Part model, mm, in its own coordinate system. Face numbers are marked on the shaded views. A direction names the side the tool comes from. Give positions to 0.01 mm unless a question says otherwise; leave off trailing zeros. Write each loop counter-clockwise with the first axis right and the second up, starting at its lowest first coordinate (ties: lowest second). Pieces come first, ordered by that corner, then holes. Notation, with made-up numbers: M 63.25,-18 L 74.25,-18 A24 cw 74.25,17 Z; hole C 46,9.25 d4. An arc over 180 degrees is marked long. Use CSV: the item, a comma, the result in double quotes. Start each with the question number.
Item 1: Cut at C-C (x = -6). List the corners of the cut face in (y, z) (3 decimals), then the cut area to 3 significant figures.
Item 2: Cut at A-A (y = 9.5). List the corners of the cut face in (x, z) (3 decimals), then the cut area to 3 significant figures.
Item 3: Cut at B-B (z = 0.6). List the corners of the cut face in (x, y) (3 decimals), then the cut area to 3 significant figures.
Item 4: Drill centre lines: line 1 (X direction, y = 2, z = 1.7) (3 decimals); line 2 (Y direction, x = 1.5, z = 0.6) (3 decimals). Where is each one in solid material? Low to high. Write a range as [from, to].
Item 5: Which spindle directions (+Z, -Z, +X, -X, +Y, -Y) get a long thin tool onto all of the face, cutting with end or side? Do the marked faces 1 and 2. Say none if no direction does.
Item 6: Pin check, flat tip, straight feed: pin 1 (0.9 mm diameter, centred on x = 5.5, z = 2.5, fed in from +Y) (3 decimals). Stop position of the tip, or through.
from build123d import *

# Parameters (mm, degrees)
F0_W     = 36.83
F0_H     = 36.83
F1_DEPTH = 3.1496
F2_W     = 31.75
F2_H     = 31.75
F3_DEPTH = 25.4
F4_W     = 31.75
F4_H     = 2.54
F5_DEPTH = 25.4


with BuildPart() as f1:
    # F0 (on Top) → F1 (new body)
    with BuildSketch(Plane.XY):
        Rectangle(F0_W, F0_H)
    extrude(amount=F1_DEPTH)

    # F2 (on face) → F3 (cut)
    with BuildSketch(Plane.XY.offset(3.1496)):
        Rectangle(F2_W, F2_H)
    extrude(amount=-F3_DEPTH, mode=Mode.SUBTRACT)

    # F4 (on face) → F5 (cut)
    with BuildSketch(Plane.XY.offset(3.1496)):
        with Locations((0, 17.145)):
            Rectangle(F4_W, F4_H)
    extrude(amount=-F5_DEPTH, mode=Mode.SUBTRACT)


solid = f1.part
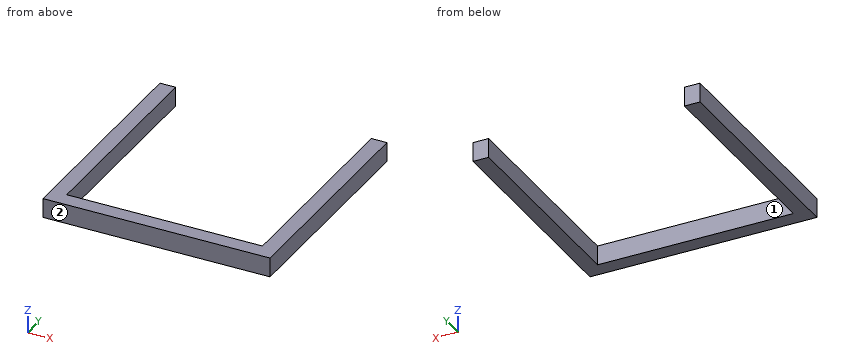
Worked answers:
1,outline,"M -18.415,0 L -15.875,0 L -15.875,3.15 L -18.415,3.15 Z"
1,area,"8.00 mm^2"
2,outline,"M -18.415,0 L -15.875,0 L -15.875,3.15 L -18.415,3.15 Z; M 15.875,0 L 18.415,0 L 18.415,3.15 L 15.875,3.15 Z"
2,area,"16.0 mm^2"
3,outline,"M -18.415,-18.415 L 18.415,-18.415 L 18.415,18.415 L 15.875,18.415 L 15.875,-15.875 L -15.875,-15.875 L -15.875,18.415 L -18.415,18.415 Z"
3,area,"268 mm^2"
4,line 1,"x = [-18.415, -15.875], [15.875, 18.415]"
4,line 2,"y = [-18.415, -15.875]"
5,face 1,"+Z, -Z, +Y"
5,face 2,"+Z, -Z, +X, -X, -Y"
6,pin 1,"stops at y = -15.875"
